Work out the finished part from the listing and answer in its coordinate system (mm). A direction names the side the tool comes from. Round coordinates to 2 decimals unless told otherwise and drop trailing zeros. Order: outer loops, then holes, each group sorted by start corner. A loop starts at its lowest first (then second) coordinate and runs counter-clockwise, first axis right, second up. Notation, with made-up numbers: (-5, 66.25) - (33, 66.25) arc R17 ccw to (33, 95.25) - close; hole circle Ø6 at (49, -33). An arc over 180 degrees is marked (long way). Put each result on its own line as item: value.
```python
from build123d import *

# Parameters (mm, degrees)
SKETCH1_R           = 13
BOSS_EXTRUDE1_DEPTH = 3


with BuildPart() as part:
    # Sketch1 → Boss-Extrude1 (new body)
    with BuildSketch(Plane.XY):
        with BuildLine():
            Line((125.012278301, 11.461790098), (11.264435627, 19.47723004))
            ThreePointArc((11.264435627, 19.47723004), (-22.5, 0), (11.264435627, -19.47723004))
            Line((11.264435627, -19.47723004), (125.012278301, -11.461790098))
            ThreePointArc((125.012278301, -11.461790098), (127.047433933, -12.146289706), (129.169709598, -12.472394231))
            Line((129.169709598, -12.472394231), (129.169709598, 0))
            Line((129.169709598, 0), (130.669709598, 0))
            Line((130.669709598, 0), (130.669709598, -12.482046669))
            ThreePointArc((130.669709598, -12.482046669), (142.165037481, 2.87434568), (125.012278301, 11.461790098))
        make_face()
        Circle(SKETCH1_R, mode=Mode.SUBTRACT)
    extrude(amount=BOSS_EXTRUDE1_DEPTH)


solid = part.part
```
1) For faces 1 (the flat face through (130.67, -6, 1)), 2 (the flat face through (59, 0, 3)), determine the directions among +Z, -Z, +X, -X, +Y, -Y from which every point of the face is accessible in a straight line to the end or side of a thin tool.
Findings below:
face 1: +Z, -Z, -Y
face 2: +Z, +X, -X, +Y, -Y
2) A cutting plane is placed at A-A on x = 0. Write down the section's boundary in (y, z).
Findings below:
outline: (-22.5, 0) - (-13, 0) - (-13, 3) - (-22.5, 3) - close; (13, 0) - (22.5, 0) - (22.5, 3) - (13, 3) - close
3) Given pin 1 Ø0.9 at (y, z) = (-6.5, 2) entering from -X; pin 2 Ø1.2 at (x, z) = (130, 1.5) entering from -Y; pin 3 Ø1.5 at (y, z) = (-8.5, 2) entering from +X; pin 4 Ø1 at (x, y) = (24.5, 8) entering from -Z, each flat-ended and moving along its own axis, determine where each tip first touches the part or whether it passes through.
Findings below:
pin 1: stops at x = -21.67
pin 2: stops at y = 0
pin 3: stops at x = 139.81
pin 4: stops at z = 0
4) A cutting plane is placed at C-C on y = -8. Write down the section's boundary in (x, z).
Findings below:
outline: (-21.03, 0) - (-10.25, 0) - (-10.25, 3) - (-21.03, 3) - close; (10.25, 0) - (129.17, 0) - (129.17, 3) - (10.25, 3) - close; (130.67, 0) - (139.6, 0) - (139.6, 3) - (130.67, 3) - close
5) Straight lines are drawn through the part: L1, parallel to X at y = -2.5, z = 0.8; L2, parallel to Y at x = 1.5, z = 2.25; L3, parallel to Y at x = -14.5, z = 2.5. For each, find the intervals that lie inside material, in ascending order. Write a range as from..to.
Findings below:
L1: x = -22.36..-12.76, 12.76..129.17, 130.67..142.25
L2: y = -22.45..-12.91, 12.91..22.45
L3: y = -17.2..17.2
6) For a pull along Y with two mould halves and no side action, classify faces 3 (the cylindrical face through (-10.316, -7.91, 1.479)), 4 (the cylindrical face through (127.02, -12.14, 1.48)), 5 (the flat face through (68.935, 15.413, 1.479)), 6 (the flat face through (129.17, -6, 1)) as pulls with the +Y half, pulls with the -Y half, needs draft (parallel to the pull), parting line crosses it, or undercut.
Findings below:
face 3: undercut
face 4: pulls with the -Y half
face 5: pulls with the +Y half
face 6: needs draft
7) A cutting plane is placed at D-D on y = 1.5. Write down the section's boundary in (x, z), then the cut area to 3 significant figures.
Findings below:
outline: (-22.45, 0) - (-12.91, 0) - (-12.91, 3) - (-22.45, 3) - close; (12.91, 0) - (142.41, 0) - (142.41, 3) - (12.91, 3) - close
area: 417 mm2
8) A cutting plane is placed at B-B on z = 0.95. Write down the section's boundary in (x, y).
Findings below:
outline: (11.26, -19.48) - (125.01, -11.46) arc R12.5 ccw to (129.17, -12.47) - (129.17, 0) - (130.67, 0) - (130.67, -12.48) arc R12.5 ccw (long way) to (125.01, 11.46) - (11.26, 19.48) arc R22.5 ccw (long way) to start; hole circle Ø26 at (0, 0)
